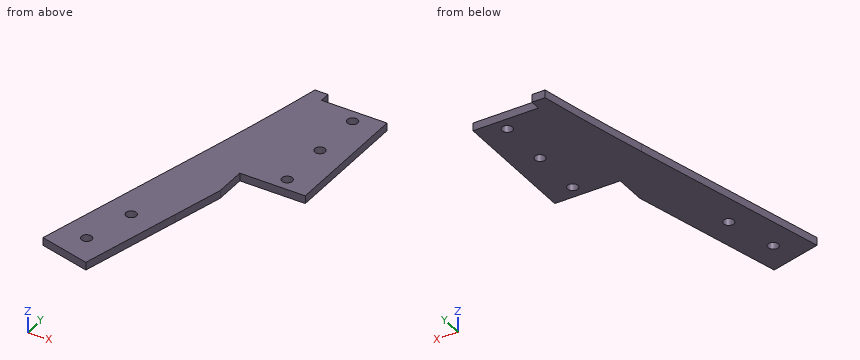
```python
from build123d import *

# Parameters (mm, degrees)
SKETCH_1_R      = 2
SKETCH_1_W      = 5
SKETCH_1_H      = 4
EXTRUDE_1_DEPTH = 3
FILLET_3_R      = 1000


with BuildPart() as part:
    # 草图1 → 凸台-拉伸1 (new body)
    # profile 1 of 2: a face of its own
    with BuildSketch(Plane.XY):
        Polygon((124.141229584, 470), (125, 470), (148, 470), (148, 520), (123, 520), (118, 520), (88.81515415, 404.428010432), (108.206427567, 399.531224216), (118, 438.31377105), (123, 458.11377105), (123, 470), align=None)
        with Locations((100.959183966, 411.675254033)):
            Circle(SKETCH_1_R, mode=Mode.SUBTRACT)
        with Locations((105.855970183, 431.06652745)):
            Circle(SKETCH_1_R, mode=Mode.SUBTRACT)
        with Locations((138, 475)):
            Circle(SKETCH_1_R, mode=Mode.SUBTRACT)
        with Locations((138, 495)):
            Circle(SKETCH_1_R, mode=Mode.SUBTRACT)
        with Locations((138, 515)):
            Circle(SKETCH_1_R, mode=Mode.SUBTRACT)
    # profile 2 of 2: a face of its own
    with BuildSketch(Plane.XY):
        with Locations((120.5, 522)):
            Rectangle(SKETCH_1_W, SKETCH_1_H)
    extrude(amount=EXTRUDE_1_DEPTH)

    # 圆角3
    # the kernel refuses this fillet: 1000 mm, written as the material it adds along each edge
    with BuildSketch(Plane(origin=(118, 520, 0), x_dir=(-0.24483931082618016, -0.9695636708716768, 0), z_dir=(0, 0, 1))) as fillet_3_piece_1:
        with BuildLine():
            CenterArc((40.368274514, -1000), FILLET_3_R, 90, 2.535967308)
            Line((-3.878254683, -0.979357243), (0, 0))
            Line((0, 0), (40.368274514, 0))
        make_face()
    extrude(amount=3)


solid = part.part
```
Check sheet for the modelled part. Datum: model origin and axes. Units: mm. Round coordinates to 2 decimals unless told otherwise and drop trailing zeros. Loops run counter-clockwise (first coordinate to the right, second up) from the corner with the lowest first, then second, coordinate; pieces in that order, holes last. Notation, with made-up numbers: (-7.5, 40) -> (8.5, 40) arc R17 cw to (8.5, 56) -> close; hole circle Ø2 at (76.25, -29.75). An arc over 180 degrees is marked (long way). Write item = value, one per line. Start each with the question number.
1) Sectioned sample at B-B, the plane y = 495. Record the cut outline in (x, z), plus the area to 3 significant figures.
2) Sectioned sample at A-A, the plane x = 138. Record the cut outline in (y, z).
3) Gauge pin test, flat ends, axial feed: pin 1 Ø0.9 at (y, z) = (521.5, 2) entering from +X; pin 2 Ø1.5 at (x, z) = (107, 1.5) entering from -Y; pin 3 Ø3.5 at (x, y) = (138, 475) entering from +Z; pin 4 Ø1.5 at (x, z) = (136, 2) entering from -Y. Record the tip position at first contact, or that the pin passes through.
4) Sectioned sample at D-D, the plane y = 515. Record the cut outline in (x, z).
5) Thickness scan on probe 1 along Y at (x, z) = (137, 1.75); probe 2 along X at (y, z) = (474, 1.65); probe 3 along Y at (x, z) = (134, 1). Record the ranges inside material, lowest first.
6) Sectioned sample at C-C, the plane z = 2.2. Record the cut outline in (x, y).
Results are:
q1.outline = (111.58, 0) -> (136, 0) -> (136, 3) -> (111.58, 3) -> close; (140, 0) -> (148, 0) -> (148, 3) -> (140, 3) -> close
q1.area = 97.3 mm^2
q2.outline = (470, 0) -> (473, 0) -> (473, 3) -> (470, 3) -> close; (477, 0) -> (493, 0) -> (493, 3) -> (477, 3) -> close; (497, 0) -> (513, 0) -> (513, 3) -> (497, 3) -> close; (517, 0) -> (520, 0) -> (520, 3) -> (517, 3) -> close
q3.pin_1 = 123
q3.pin_2 = 399.65
q3.pin_3 = through
q3.pin_4 = 470
q4.outline = (116.1, 0) -> (136, 0) -> (136, 3) -> (116.1, 3) -> close; (140, 0) -> (148, 0) -> (148, 3) -> (140, 3) -> close
q5.probe_1 = 470 to 473.27, 476.73 to 493.27, 496.73 to 513.27, 516.73 to 520
q5.probe_2 = 106.38 to 136.27, 139.73 to 148
q5.probe_3 = 470 to 520
q6.outline = (88.82, 404.43) -> (108.21, 399.53) -> (123, 458.11) -> (123, 470) -> (148, 470) -> (148, 520) -> (123, 520) -> (123, 524) -> (118, 524) arc R1000 cw to (108.12, 480.86) -> close; hole circle Ø4 at (100.96, 411.68); hole circle Ø4 at (105.86, 431.07); hole circle Ø4 at (138, 475); hole circle Ø4 at (138, 495); hole circle Ø4 at (138, 515)
